Could you check a few things on this drawing? It's one solid part, dimensions in mm from its lowest x, y, z. A direction names the side the tool comes from. Give positions to 0.01 mm unless a question says otherwise; leave off trailing zeros. Order: outer loops, then holes, each group sorted by start corner. A loop starts at its lowest first (then second) coordinate and runs counter-clockwise, first axis right, second up. Notation, with made-up numbers: (11.25, 82.5) - (47.25, 82.5) arc R22 ccw to (47.25, 88.5) - close; hole circle Ø10 at (-31, 41.5). An arc over 180 degrees is marked (long way). Return JSON: item names as keys, results as strings.
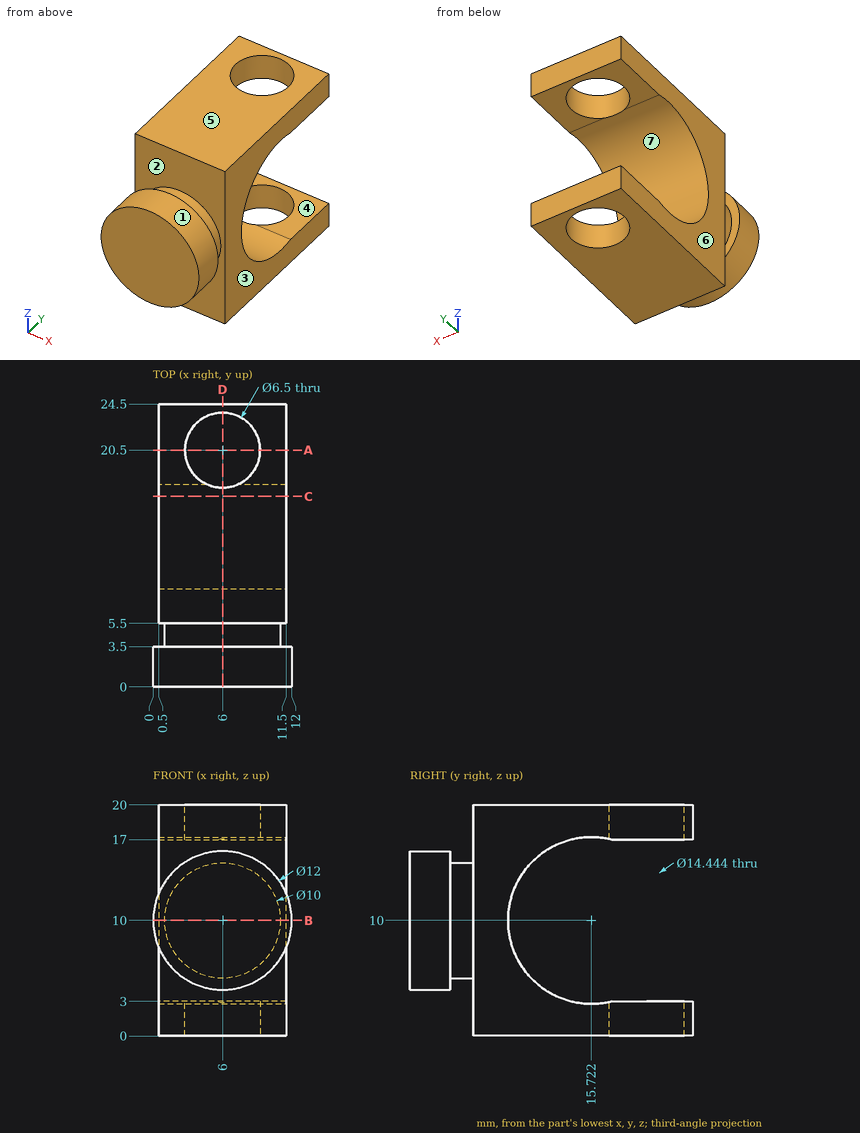
1. Suppose I cut it at C-C (y = 16.5). List the corners of the cut face in (x, z) for me.
Checks:
{"outline": "(0.5, 0) - (11.5, 0) - (11.5, 2.82) - (0.5, 2.82) - close; (0.5, 17.18) - (11.5, 17.18) - (11.5, 20) - (0.5, 20) - close"}
2. If I drill on L1, parallel to Z at x = 11, y = 17.5; L2, parallel to X at y = 20.5, z = 1.3; L3, parallel to Y at x = 6, z = 18.25, over which ranges is the centre line in solid material (lowest first)? Write a range as [from, to].
Checks:
{"L1": "[0, 3], [17, 20]", "L2": "[0.5, 2.75], [9.25, 11.5]", "L3": "[5.5, 17.25], [23.75, 24.5]"}
3. On a 3-axis mill with a long thin cutter (end or side, diameter ignored), from which of +Z, -Z, +X, -X, +Y, -Y can I reach the whole of each face in a straight line? I mean the marked faces 1, 2, 3 and 4. Say none if no direction works.
Checks:
{"face 1": "-Y", "face 2": "none", "face 3": "+Z, -Z, +X, +Y", "face 4": "+X, -X, +Y"}
4. Thinking about a two-plate mould opening in Z: for the marked faces 5, 6 and 7, which applies, +Z half, -Z half, draft (parallel to the pull), parting line (faces both ways), or undercut?
Checks:
{"face 5": "+Z half", "face 6": "draft", "face 7": "undercut"}
5. Suppose I cut it at D-D (x = 6). State how many separate pieces and enclosed holes the cut face has, plus the area to 3 significant figures.
Checks:
{"separate pieces": "3", "enclosed holes": "0", "area": "198 mm^2"}
6. Suppose I cut it at B-B (z = 10). List the corners of the cut face in (x, y) for me, plus the area to 3 significant figures.
Checks:
{"outline": "(0, 0) - (12, 0) - (12, 3.5) - (11, 3.5) - (11, 5.5) - (11.5, 5.5) - (11.5, 8.5) - (0.5, 8.5) - (0.5, 5.5) - (1, 5.5) - (1, 3.5) - (0, 3.5) - close", "area": "95.0 mm^2"}
7. Suppose I cut it at A-A (y = 20.5). List the corners of the cut face in (x, z) for me, plus the area to 3 significant figures.
Checks:
{"outline": "(0.5, 0) - (2.75, 0) - (2.75, 3) - (0.5, 3) - close; (0.5, 17) - (2.75, 17) - (2.75, 20) - (0.5, 20) - close; (9.25, 0) - (11.5, 0) - (11.5, 3) - (9.25, 3) - close; (9.25, 17) - (11.5, 17) - (11.5, 20) - (9.25, 20) - close", "area": "27.0 mm^2"}
8. For pin 1 Ø4 at (y, z) = (10, 12.5) entering from -X; pin 2 Ø6 at (x, z) = (4, 12.5) entering from +Y; pin 3 Ø3.5 at (x, y) = (6, 20) entering from -Z; pin 4 Ø5.5 at (y, z) = (11.5, 14.5) entering from +X, each with a flat end and sliding along its axis, tell me the tip position at first contact or that it passes through.
Checks:
{"pin 1": "x = 0.5", "pin 2": "y = 11.04", "pin 3": "through", "pin 4": "x = 11.5"}
